Can you work these out from the model? Positions are in its coordinate system, mm. A direction names the side the tool comes from. Give positions to 0.01 mm unless a question says otherwise; leave off trailing zeros. Answer as CSV lines item,"result".
```python
from build123d import *


with BuildPart() as part:
    # Sketch5 → Loft11 section 0
    with BuildSketch(Plane(origin=(0, 43.994090512, 0), x_dir=(1, 0, 0), z_dir=(0, 1, 0))):
        with BuildLine():
            Line((76.2, 0.048006), (76.2, -0.048006))
            add(Edge.make_bspline(
                [(76.2, -0.048006), (76.192583251, -0.049047765), (76.162942912, -0.053211081), (76.044647253, -0.069755857), (75.867562125, -0.094486743), (75.632052521, -0.126965392), (75.390396557, -0.160190201), (75.106127116, -0.198904989), (74.779917937, -0.242859006), (74.412541545, -0.291864294), (74.004851816, -0.345569023), (73.55779868, -0.403720926), (73.072416984, -0.465853222), (72.352060102, -0.55677244), (71.584541596, -0.651127112), (70.771637318, -0.748448048), (70.113353772, -0.825737809), (69.424771293, -0.904853153), (68.707537282, -0.985592031), (67.963304352, -1.067375261), (67.193834288, -1.14998319), (66.400894079, -1.232825488), (65.586352847, -1.315748636), (64.752102975, -1.398113207), (63.90010602, -1.479660513), (63.032340473, -1.559824173), (62.150830619, -1.638342101), (61.257640656, -1.714565201), (60.354852072, -1.788152536), (59.444584786, -1.858634165), (58.528953151, -1.925444296), (57.610108942, -1.988163902), (56.690197069, -2.046291991), (55.467880801, -2.116763144), (54.251069434, -2.176215597), (52.748712156, -2.234066929), (51.565971548, -2.266645454), (50.400091132, -2.283584551), (49.548035029, -2.288048273), (48.713726655, -2.284102235), (47.899118606, -2.271569022), (47.10611977, -2.250069868), (46.336564553, -2.21969991), (45.59224861, -2.180240934), (44.874904805, -2.131803537), (44.186222319, -2.074397819), (43.527802298, -2.008128116), (42.901174603, -1.933245819), (42.307783855, -1.850055304), (41.749027942, -1.758711647), (41.226187427, -1.659671366), (40.740465618, -1.55330687), (40.292997688, -1.439978722), (39.8847724, -1.320194614), (39.516689892, -1.194352348), (39.189535118, -1.062886557), (38.903955697, -0.926176493), (38.660495695, -0.784506781), (38.45943861, -0.638117579), (38.30117294, -0.486768084), (38.186080347, -0.330029549), (38.115712554, -0.167135854), (38.092341043, 0), (38.115712554, 0.167135854), (38.186080347, 0.330029549), (38.30117294, 0.486768084), (38.45943861, 0.638117579), (38.660495695, 0.784506781), (38.903955697, 0.926176493), (39.189535118, 1.062886557), (39.516689892, 1.194352348), (39.8847724, 1.320194614), (40.292997688, 1.439978722), (40.740465618, 1.55330687), (41.226187427, 1.659671366), (41.749027942, 1.758711647), (42.307783855, 1.850055304), (42.901174603, 1.933245819), (43.527802298, 2.008128116), (44.186222319, 2.074397819), (44.874904805, 2.131803537), (45.59224861, 2.180240934), (46.336564553, 2.21969991), (47.10611977, 2.250069868), (47.899118606, 2.271569022), (48.713726655, 2.284102235), (49.548035029, 2.288048273), (50.400091132, 2.283584551), (51.565971548, 2.266645454), (53.052575769, 2.225697023), (54.554732583, 2.162253193), (55.771346838, 2.09926718), (56.690197069, 2.046291991), (57.610108942, 1.988163902), (58.528953151, 1.925444296), (59.444584786, 1.858634165), (60.354852072, 1.788152536), (61.257640656, 1.714565201), (62.150830619, 1.638342101), (63.032340473, 1.559824173), (63.90010602, 1.479660513), (64.752102975, 1.398113207), (65.586352847, 1.315748636), (66.400894079, 1.232825488), (67.193834288, 1.14998319), (67.963304352, 1.067375261), (68.707537282, 0.985592031), (69.424771293, 0.904853153), (70.113353772, 0.825737809), (70.771637318, 0.748448048), (71.584541596, 0.651127112), (72.352060102, 0.55677244), (73.072416984, 0.465853222), (73.55779868, 0.403720926), (74.004851816, 0.345569023), (74.412541545, 0.291864294), (74.779917937, 0.242859006), (75.106127116, 0.198904989), (75.390396557, 0.160190201), (75.632052521, 0.126965392), (75.867562125, 0.094486743), (76.044647253, 0.069755857), (76.162942912, 0.053211081), (76.192583251, 0.049047765), (76.2, 0.048006)],
                knots=[0, 0, 0, 0, 0.000289201, 0.001155766, 0.004612322, 0.007193518, 0.010335793, 0.014031397, 0.018271612, 0.023045847, 0.028342901, 0.03415012, 0.04045376, 0.04723833, 0.062186613, 0.070313724, 0.078851908, 0.087780126, 0.097077521, 0.106722049, 0.116690868, 0.126960505, 0.137507218, 0.148306055, 0.159330765, 0.17055649, 0.181956531, 0.193504043, 0.205171367, 0.2169323, 0.228758169, 0.2406214, 0.252494936, 0.264350287, 0.287897994, 0.299535854, 0.322404759, 0.333584032, 0.344559266, 0.35530596, 0.365799778, 0.37601757, 0.3859373, 0.395537659, 0.404797976, 0.413698812, 0.422221441, 0.430349273, 0.438066019, 0.445356904, 0.452209372, 0.458611567, 0.464554044, 0.47002985, 0.475034902, 0.479569141, 0.483636857, 0.487250263, 0.490431338, 0.493218828, 0.495674086, 0.497891368, 0.5, 0.502108632, 0.504325914, 0.506781172, 0.509568662, 0.512749737, 0.516363143, 0.520430859, 0.524965098, 0.52997015, 0.535445956, 0.541388433, 0.547790628, 0.554643096, 0.561933981, 0.569650727, 0.577778559, 0.586301188, 0.595202024, 0.604462341, 0.6140627, 0.62398243, 0.634200222, 0.64469404, 0.655440734, 0.666415968, 0.677595241, 0.700464146, 0.723839427, 0.735649713, 0.747505064, 0.7593786, 0.771241831, 0.7830677, 0.794828633, 0.806495957, 0.818043469, 0.82944351, 0.840669235, 0.851693945, 0.862492782, 0.873039495, 0.883309132, 0.893277951, 0.902922479, 0.912219874, 0.921148092, 0.929686276, 0.937813387, 0.95276167, 0.95954624, 0.96584988, 0.971657099, 0.976954153, 0.981728388, 0.985968603, 0.989664207, 0.992806482, 0.995387678, 0.998844234, 0.999710799, 1, 1, 1, 1], degree=3))
        make_face()
    # Sketch3 → Loft11 section 1
    with BuildSketch(Plane(origin=(0, 0, 0), x_dir=(1, 0, 0), z_dir=(0, 1, 0))):
        with BuildLine():
            Line((76.2, 0.096012), (76.2, -0.096012))
            add(Edge.make_bspline(
                [(76.2, -0.096012), (76.185166502, -0.09809553), (76.125885823, -0.106422162), (75.889294507, -0.139511713), (75.53512425, -0.188973486), (75.064105041, -0.253930784), (74.580793115, -0.320380401), (74.012254232, -0.397809978), (73.359835874, -0.485718012), (72.62508309, -0.583728588), (71.809703632, -0.691138045), (70.915597359, -0.807441851), (69.944833968, -0.931706445), (68.504120203, -1.113544881), (66.969083191, -1.302254225), (65.343274636, -1.496896097), (64.026707544, -1.651475618), (62.649542587, -1.809706305), (61.215074564, -1.971184062), (59.726608705, -2.134750522), (58.187668577, -2.299966381), (56.601788159, -2.465650976), (54.972705694, -2.631497273), (53.30420595, -2.796226414), (51.60021204, -2.959321026), (49.864680946, -3.119648346), (48.101661238, -3.276684202), (46.315281313, -3.429130403), (44.509704144, -3.576305072), (42.689169571, -3.71726833), (40.857906302, -3.850888591), (39.020217884, -3.976327805), (37.180394137, -4.092583982), (34.735761601, -4.233526287), (32.302138868, -4.352431193), (29.297424312, -4.468133858), (26.931943095, -4.533290908), (24.600182263, -4.567169102), (22.896070057, -4.576096546), (21.22745331, -4.56820447), (19.598237213, -4.543138044), (18.01223954, -4.500139735), (16.473129105, -4.43939982), (14.98449722, -4.360481867), (13.549809609, -4.263607073), (12.172444638, -4.148795638), (10.855604596, -4.016256231), (9.602349205, -3.866491638), (8.41556771, -3.700110609), (7.298055884, -3.517423293), (6.252374854, -3.319342733), (5.280931237, -3.10661374), (4.385995376, -2.879957444), (3.569544801, -2.640389227), (2.833379783, -2.388704697), (2.179070236, -2.125773113), (1.607911394, -1.852352986), (1.120991389, -1.569013562), (0.71887722, -1.276235157), (0.40234588, -0.973536168), (0.172160694, -0.660059098), (0.031425108, -0.334271708), (-0.015317913, 0), (0.031425108, 0.334271708), (0.172160694, 0.660059098), (0.40234588, 0.973536168), (0.71887722, 1.276235157), (1.120991389, 1.569013562), (1.607911394, 1.852352986), (2.179070236, 2.125773113), (2.833379783, 2.388704697), (3.569544801, 2.640389227), (4.385995376, 2.879957444), (5.280931237, 3.10661374), (6.252374854, 3.319342733), (7.298055884, 3.517423293), (8.41556771, 3.700110609), (9.602349205, 3.866491638), (10.855604596, 4.016256231), (12.172444638, 4.148795638), (13.549809609, 4.263607073), (14.98449722, 4.360481867), (16.473129105, 4.43939982), (18.01223954, 4.500139735), (19.598237213, 4.543138044), (21.22745331, 4.56820447), (22.896070057, 4.576096546), (24.600182263, 4.567169102), (26.931943095, 4.533290908), (29.905151537, 4.451394045), (32.909465167, 4.324506385), (35.342693676, 4.198534359), (37.180394137, 4.092583982), (39.020217884, 3.976327805), (40.857906302, 3.850888591), (42.689169571, 3.71726833), (44.509704144, 3.576305072), (46.315281313, 3.429130403), (48.101661238, 3.276684202), (49.864680946, 3.119648346), (51.60021204, 2.959321026), (53.30420595, 2.796226414), (54.972705694, 2.631497273), (56.601788159, 2.465650976), (58.187668577, 2.299966381), (59.726608705, 2.134750522), (61.215074564, 1.971184062), (62.649542587, 1.809706305), (64.026707544, 1.651475618), (65.343274636, 1.496896097), (66.969083191, 1.302254225), (68.504120203, 1.113544881), (69.944833968, 0.931706445), (70.915597359, 0.807441851), (71.809703632, 0.691138045), (72.62508309, 0.583728588), (73.359835874, 0.485718012), (74.012254232, 0.397809978), (74.580793115, 0.320380401), (75.064105041, 0.253930784), (75.53512425, 0.188973486), (75.889294507, 0.139511713), (76.125885823, 0.106422162), (76.185166502, 0.09809553), (76.2, 0.096012)],
                knots=[0, 0, 0, 0, 0.000289201, 0.001155766, 0.004612322, 0.007193518, 0.010335793, 0.014031397, 0.018271612, 0.023045847, 0.028342901, 0.03415012, 0.04045376, 0.04723833, 0.062186613, 0.070313724, 0.078851908, 0.087780126, 0.097077521, 0.106722049, 0.116690868, 0.126960505, 0.137507218, 0.148306055, 0.159330765, 0.17055649, 0.181956531, 0.193504043, 0.205171367, 0.2169323, 0.228758169, 0.2406214, 0.252494936, 0.264350287, 0.287897994, 0.299535854, 0.322404759, 0.333584032, 0.344559266, 0.35530596, 0.365799778, 0.37601757, 0.3859373, 0.395537659, 0.404797976, 0.413698812, 0.422221441, 0.430349273, 0.438066019, 0.445356904, 0.452209372, 0.458611567, 0.464554044, 0.47002985, 0.475034902, 0.479569141, 0.483636857, 0.487250263, 0.490431338, 0.493218828, 0.495674086, 0.497891368, 0.5, 0.502108632, 0.504325914, 0.506781172, 0.509568662, 0.512749737, 0.516363143, 0.520430859, 0.524965098, 0.52997015, 0.535445956, 0.541388433, 0.547790628, 0.554643096, 0.561933981, 0.569650727, 0.577778559, 0.586301188, 0.595202024, 0.604462341, 0.6140627, 0.62398243, 0.634200222, 0.64469404, 0.655440734, 0.666415968, 0.677595241, 0.700464146, 0.723839427, 0.735649713, 0.747505064, 0.7593786, 0.771241831, 0.7830677, 0.794828633, 0.806495957, 0.818043469, 0.82944351, 0.840669235, 0.851693945, 0.862492782, 0.873039495, 0.883309132, 0.893277951, 0.902922479, 0.912219874, 0.921148092, 0.929686276, 0.937813387, 0.95276167, 0.95954624, 0.96584988, 0.971657099, 0.976954153, 0.981728388, 0.985968603, 0.989664207, 0.992806482, 0.995387678, 0.998844234, 0.999710799, 1, 1, 1, 1], degree=3))
        make_face()
    loft()

    # Sketch8 → Cut-Revolve1 (revolve, cut)
    with BuildSketch(Plane.XY, mode=Mode.PRIVATE) as cut_revolve1_sk:
        Polygon((20.955, 0), (20.955, 12.7), (19.05, 15.999556788), (19.05, 0), align=None)
    cut_revolve1 = revolve(cut_revolve1_sk.sketch.rotate(Axis((19.05, 15.999556788, 0), (0, -1, 0)), 180), axis=Axis((19.05, 15.999556788, 0), (0, -1, 0)), mode=Mode.SUBTRACT)

    # Mirror1: Cut-Revolve1 across plane
    add(cut_revolve1.mirror(Plane(origin=(22.225, 0, 0), x_dir=(0, 0, 1), z_dir=(1, 0, 0))), mode=Mode.SUBTRACT)

    # Mirror2: Cut-Revolve1 across plane
    add(cut_revolve1.mirror(Plane(origin=(28.575, 0, 0), x_dir=(0, 0, 1), z_dir=(1, 0, 0))), mode=Mode.SUBTRACT)

    # Mirror2 copy 1 sketch → Mirror2 copy 1 (revolve, cut)
    with BuildSketch(Plane(origin=(12.7, 0, 0), x_dir=(1, 0, 0), z_dir=(0, 0, 1))):
        Polygon((20.955, 0), (20.955, 12.7), (19.05, 15.999556788), (19.05, 0), align=None)
    revolve(axis=Axis((31.75, 15.999556788, 0), (0, -1, 0)), mode=Mode.SUBTRACT)


solid = part.part
```
1) Which directions (+Z, -Z, +X, -X, +Y, -Y) give clear straight access to the entire face, cutting with the end or side of a thin tool? Please do faces 1 (the cylindrical face through (29.847, 6.439, 0.084)), 2 (the flat face through (53, 43.994, 0)).
Answer block:
face 1,"-Y"
face 2,"+Z, -Z, +X, -X, +Y"
2) I need wall thicknesses on line 1 along Z through (x, y) = (57, 39.5); line 2 along Z through (x, y) = (35, 24.5); line 3 along Y through (x, z) = (26.5, -0.25). Which ranges of each line are inside material? Lowest first, please. Write a range as [from, to].
Answer block:
line 1,"[-2.1, 2.1]"
line 2,"[-3.27, 3.27]"
line 3,"[14.05, 30.55]"
3) I'm going to push flat-ended pins straight in: P1, Ø8, axis at x = 22, y = 35, coming from the -Z side; P2, Ø2, axis at y = 34.5, z = 0, coming from the -X side; P3, Ø1, axis at x = 46.5, y = 21.5, coming from the -Z side; P4, Ø1, axis at x = 16.5, y = 15, coming from the -Z side. Where does each tip first touch, or does it pass through?
Answer block:
P1,"through"
P2,"x = 29.01"
P3,"z = -3.14"
P4,"z = -2.53"
4) If we mould it in two halves opening along X, with no side actions, what happens to faces 3 (the conical face through (19.8, 14.7, 0)), 4 (the flat face through (30, 0, -2))? For each: +X half, -X half, draft (parallel to the pull), parting line (faces both ways), or undercut.
Answer block:
face 3,"undercut"
face 4,"draft"
